For this review, take the finished solid that the model builds, in its own axes (mm). Face numbers are marked on the shaded views. A direction names the side the tool comes from. Give positions to 0.01 mm unless a question says otherwise; leave off trailing zeros. Order: outer loops, then holes, each group sorted by start corner. A loop starts at its lowest first (then second) coordinate and runs counter-clockwise, first axis right, second up. Notation, with made-up numbers: (3, -39.75) - (18, -39.75) arc R22 ccw to (18, -33.75) - close; hole circle Ø3 at (-3.75, 74). An arc over 180 degrees is marked (long way). Use a Markdown table: item, result. Add a question column.
1) Mouldability with a two-part tool opening along X and no side actions: class the marked faces 1, 2 and 3 as released by +X, released by -X, zero draft, split by the parting line, or undercut.
2) We need section B-B on y = -14.5. Write out the cut boundary in (x, z).
3) Clearance check with a flat-ended pin moving along its axis: P1, Ø4, axis at x = -4.5, y = 5, coming from the +Z side. State where the tip first meets the part, or that it passes through.
4) Machinability: for the marked faces 4, 5 and 6, which of the approach directions +Z, -Z, +X, -X, +Y, -Y give a long, thin tool a straight path to every point of the face, cutting with its end or side? Answer none if there is none.
5) Wall thickness on L1, parallel to X at y = 4.5, z = 7.75; L2, parallel to Y at x = -16.5, z = 4.25; L3, parallel to Y at x = 7.5, z = 2.25: over which ranges is each line inside the solid? List them lowest first.
6) We need section A-A on x = 14.5. Write out the cut boundary in (y, z).
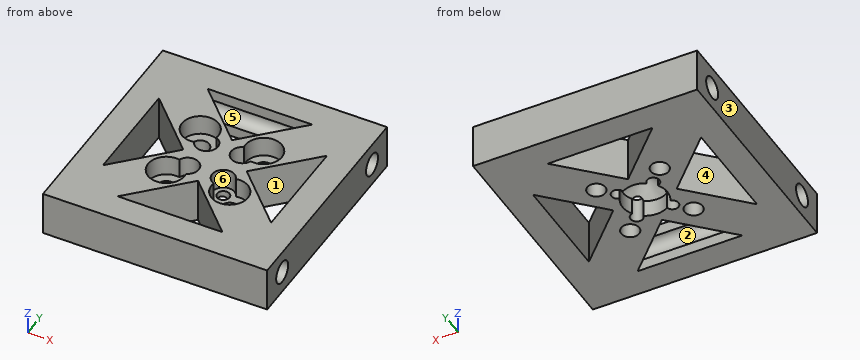
Autodesk Fusion 360 part; units mm, degrees
sketch "Sketch1" plane through (0, 0, 0) normal (0, 0, 1) x (1, 0, 0)
  line L0 (20, -20) -> (-20, -20)
  line L1 (-20, -20) -> (-20, 20)
  line L2 (-20, 20) -> (20, 20)
  line L3 (20, 20) -> (20, -20)
  line L4 (20, -20) -> (-20, 20) construction
  line L5 (-20, -20) -> (20, 20) construction
  dimension "d1" = 40
  dimension "d2" = 40
extrude "Extrude1" add sketch "Sketch1" along normal blind 8
sketch "Sketch2" plane through (20, 0, 0) normal (1, 0, 0) x (0, 1, 0)
  line L0 (-20, 0) -> (20, 0)
  line L1 (20, 0) -> (20, 8)
  line L2 (20, 8) -> (-20, 8)
  line L3 (-20, 8) -> (-20, 0)
  line L4 (-20, 4) -> (20, 4) construction
  line L5 (0, 8) -> (0, 0) construction
  point P0 (-15, 4)
  point P1 (15, 4)
  point P2 (-20, 4)
  point P3 (20, 4)
  dimension "d5" = 30
sketch "Sketch3" plane through (0, 0, 8) normal (0, 0, 1) x (-1, 0, 0)
  line L0 (-20, -20) -> (20, -20)
  line L1 (20, -20) -> (20, 20)
  line L2 (20, 20) -> (-20, 20)
  line L3 (-20, 20) -> (-20, -20)
  line L4 (-20, -20) -> (-20, 20)
  line L5 (-20, 20) -> (20, 20)
  line L6 (20, -20) -> (-20, -20)
  line L7 (20, 20) -> (20, -20)
  line L8 (-15, 15) -> (-15, -15)
  line L9 (-15, -15) -> (15, -15)
  line L10 (15, -15) -> (15, 15)
  line L11 (15, 15) -> (-15, 15)
  line L12 (15, 15) -> (-15, -15) construction
  line L13 (-15, 15) -> (15, -15) construction
  line L14 (9.3431, -15) -> (-15, 9.3431)
  line L15 (15, -9.3431) -> (-9.3431, 15)
  line L16 (9.3431, 15) -> (-15, -9.3431)
  line L17 (-9.3431, -15) -> (15, 9.3431)
  point P0 (5.6569, -5.6569)
  point P1 (-5.6569, 5.6569)
  point P2 (-5.6569, -5.6569)
  point P3 (5.6569, 5.6569)
  point P4 (3.182, 3.182)
  point P5 (-3.182, 3.182)
  point P6 (-3.182, -3.182)
  point P7 (3.182, -3.182)
  dimension "d24" = -5
  dimension "d25" = 8
  dimension "d26" = 8
  dimension "d49" = 16
  dimension "d50" = 9
extrude "Extrude3" cut sketch "Sketch3" against normal up to surface (8 mm away) contours L8 L14 L16 | L11 L15 L16 | L9 L14 L17 | L10 L15 L17
hole "Hole2" at (20, -15, 4) at (20, 15, 4) direction (-1, 0, 0) diameter 4 end up to surface (40 mm away)
hole "Hole3" at (-5.6569, 5.6569, 8) at (5.6569, 5.6569, 8) at (5.6569, -5.6569, 8) at (-5.6569, -5.6569, 8) direction (0, 0, -1) diameter 3.2 end up to surface (8 mm away) counterbore diameter 6.5 counterbore depth 3.6
hole "Hole4" at (-3.182, 3.182, 8) at (3.182, 3.182, 8) at (3.182, -3.182, 8) at (-3.182, -3.182, 8) direction (0, 0, -1) diameter 2.2 end up to surface (8 mm away) counterbore diameter 4 counterbore depth 3.6
sketch "Sketch5" plane through (0, 0, 0) normal (0, 0, 1) x (1, 0, 0)
hole "Hole6" at (0, 0, 0) direction (0, 0, 1) diameter 8 depth 3 tip angle 118
equation "d26 = d25"
Checked values:
| question | item | result |
|---|---|---|
| 1 | face 1 | undercut |
| 1 | face 2 | zero draft |
| 1 | face 3 | released by -X |
| 2 | outline | (-20, 0) - (-8.84, 0) - (-8.84, 2.06) - (-20, 2.06) - close; (-20, 5.94) - (-8.84, 5.94) - (-8.84, 8) - (-20, 8) - close; (8.84, 0) - (20, 0) - (20, 2.06) - (8.84, 2.06) - close; (8.84, 5.94) - (20, 5.94) - (20, 8) - (8.84, 8) - close |
| 3 | P1 | z = 4.4 |
| 4 | face 4 | +Z, -Z |
| 4 | face 5 | +X, -X |
| 4 | face 6 | +Z |
| 5 | L1 | -20 to -15, -10.16 to -8.69, -1.68 to 1.68, 8.69 to 10.16, 15 to 20 |
| 5 | L2 | -20 to -16.98, -13.02 to 13.02, 16.98 to 20 |
| 5 | L3 | -20 to -15.97, -13.16 to -1.84, 1.84 to 13.16, 15.97 to 20 |
| 6 | outline | (-20, 0) - (-8.84, 0) - (-8.84, 8) - (-20, 8) - close; (8.84, 0) - (20, 0) - (20, 8) - (8.84, 8) - close; hole circle Ø4 at (-15, 4); hole circle Ø4 at (15, 4) |
